Check sheet for the modelled part. Datum: model origin and axes. Units: mm. A direction names the side the tool comes from. Give positions to 0.01 mm unless a question says otherwise; leave off trailing zeros. Order: outer loops, then holes, each group sorted by start corner. A loop starts at its lowest first (then second) coordinate and runs counter-clockwise, first axis right, second up. Notation, with made-up numbers: (51, 10) -> (106, 10) arc R27 cw to (106, 36) -> close; hole circle Ø5 at (30, 9.5). An arc over 180 degrees is marked (long way). One line per question, with ' | ' between items.
```python
from build123d import *

# Parameters (mm, degrees)
SKETCH1_R           = 10
BOSS_EXTRUDE1_DEPTH = 10
SKETCH3_R           = 10
BOSS_EXTRUDE2_DEPTH = 10


with BuildPart() as part:
    # Sketch1 → Boss-Extrude1 (new body)
    with BuildSketch(Plane(origin=(0, 0, 0), x_dir=(1, 0, 0), z_dir=(0, 1, 0))):
        with BuildLine():
            Line((-35, 20), (35, 20))
            Line((35, 20), (35, -20))
            Line((35, -20), (-35, -20))
            ThreePointArc((-35, -20), (-55, 0), (-35, 20))
        make_face()
        with Locations(Location((-35, 0, 0), (0, 0, 270))):
            Circle(SKETCH1_R, mode=Mode.SUBTRACT)
    extrude(amount=BOSS_EXTRUDE1_DEPTH)

    # Sketch3 → Boss-Extrude2 (add)
    with BuildSketch(Plane(origin=(35, 0, 0), x_dir=(0, 0, -1), z_dir=(1, 0, 0))):
        with BuildLine():
            Line((-20, 10), (20, 10))
            Line((20, 10), (20, 30))
            ThreePointArc((20, 30), (0, 50), (-20, 30))
            Line((-20, 30), (-20, 10))
        make_face()
        with Locations((0, 30)):
            Circle(SKETCH3_R, mode=Mode.SUBTRACT)
    extrude(amount=-BOSS_EXTRUDE2_DEPTH)


solid = part.part
```
Q1. Section check D-D (y = 8). Enter the section's corners in (x, z).
Result sheet:
outline: (-35, -20) -> (35, -20) -> (35, 20) -> (-35, 20) arc R20 ccw to start; hole circle Ø20 at (-35, 0)
Q2. Thickness scan on line 1 (X direction, y = 2.5, z = 0); line 2 (Y direction, x = 30.25, z = 0); line 3 (X direction, y = 34.5, z = 18.5). Record the ranges inside material, lowest first.
Result sheet:
line 1: x = -55 to -45, -25 to 35 | line 2: y = 0 to 20, 40 to 50 | line 3: x = 25 to 35
Q3. Section check C-C (x = -42.5). Enter the section's corners in (y, z).
Result sheet:
outline: (0, -18.54) -> (10, -18.54) -> (10, -6.61) -> (0, -6.61) -> close; (0, 6.61) -> (10, 6.61) -> (10, 18.54) -> (0, 18.54) -> close
Q4. Mould release check, pull along Z, two halves, no side actions. Record for faces 1 (the face through (8, 8, -20)), 2 (the face through (8, 9, 20)), 3 (the face through (-44.76, 4.93, -2.17)): pulls with the +Z half, pulls with the -Z half, needs draft (parallel to the pull), parting line crosses it, or undercut.
Result sheet:
face 1: pulls with the -Z half | face 2: pulls with the +Z half | face 3: undercut
Q5. Section check B-B (y = 22). Enter the section's corners in (x, z), and give its area (3 significant figures).
Result sheet:
outline: (25, -20) -> (35, -20) -> (35, -6) -> (25, -6) -> close; (25, 6) -> (35, 6) -> (35, 20) -> (25, 20) -> close | area: 280 mm2
Q6. Access from +Z, -Z, +X, -X, +Y, -Y to the whole of each face (thin tool, end or side, straight path). Record for faces 4 (the face through (-14, 10, 0)), 5 (the face through (35, 19.8, 0.3)).
Result sheet:
face 4: +Z, -Z, -X, +Y | face 5: +Z, -Z, +X, +Y, -Y
Q7. Depth check by flat-ended pin: pin 1 Ø3 at (x, z) = (17.5, -12) entering from +Y; pin 2 Ø20 at (y, z) = (27, 7) entering from -X; pin 3 Ø6 at (x, y) = (-41, 8) entering from +Z. Enter the tip coordinate at first touch or a pass-through.
Result sheet:
pin 1: stops at y = 10 | pin 2: stops at x = 25 | pin 3: stops at z = 19.77
Q8. Section check A-A (z = 0). Enter the section's corners in (x, y).
Result sheet:
outline: (-55, 0) -> (-45, 0) -> (-45, 10) -> (-55, 10) -> close; (-25, 0) -> (35, 0) -> (35, 20) -> (25, 20) -> (25, 10) -> (-25, 10) -> close; (25, 40) -> (35, 40) -> (35, 50) -> (25, 50) -> close
